```python
from build123d import *

# Parameters (mm, degrees)
SKETCH_1_W          = 92
SKETCH_1_H          = 67
EXTRUDE_1_DEPTH     = 34
SKETCH_2_W          = 86
SKETCH_2_H          = 61
CUT_EXTRUDE_1_DEPTH = 3
SKETCH_3_R          = 1.5
CUT_EXTRUDE_2_DEPTH = 3
SKETCH_4_W          = 86
SKETCH_4_H          = 61
CUT_EXTRUDE_3_DEPTH = 3
SKETCH_5_R          = 1.5
CUT_EXTRUDE_4_DEPTH = 3


with BuildPart() as part:
    # 草图1 → 凸台-拉伸1 (new body)
    with BuildSketch(Plane(origin=(0, 0, 0), x_dir=(1, 0, 0), z_dir=(0, 1, 0))):
        Rectangle(SKETCH_1_W, SKETCH_1_H)
    extrude(amount=EXTRUDE_1_DEPTH)

    # 草图2 → 切除-拉伸1 (cut)
    with BuildSketch(Plane(origin=(0, 34, 0), x_dir=(1, 0, 0), z_dir=(0, 1, 0))):
        Rectangle(SKETCH_2_W, SKETCH_2_H)
    extrude(amount=-CUT_EXTRUDE_1_DEPTH, mode=Mode.SUBTRACT)

    # 草图3 → 切除-拉伸2 (cut)
    with BuildSketch(Plane(origin=(0, 31, 0), x_dir=(1, 0, 0), z_dir=(0, 1, 0))):
        with Locations(Location((25, -16.5, 0), (0, 0, 270))):
            Circle(SKETCH_3_R)
        with Locations(Location((25, -7.5, 0), (0, 0, 270))):
            Circle(SKETCH_3_R)
    extrude(amount=-CUT_EXTRUDE_2_DEPTH, mode=Mode.SUBTRACT)

    # 草图4 → 切除-拉伸3 (cut)
    with BuildSketch(Plane.XZ):
        Rectangle(SKETCH_4_W, SKETCH_4_H)
    extrude(amount=-CUT_EXTRUDE_3_DEPTH, mode=Mode.SUBTRACT)

    # 草图5 → 切除-拉伸4 (cut)
    with BuildSketch(Plane.XZ.offset(-3)):
        with Locations(Location((-39, 24.5, 0), (0, 0, 270))):
            Circle(SKETCH_5_R)
        with Locations(Location((19, 24.5, 0), (0, 0, 90))):
            Circle(SKETCH_5_R)
        with Locations(Location((19, -24.5, 0), (0, 0, 270))):
            Circle(SKETCH_5_R)
        with Locations(Location((-39, -24.5, 0), (0, 0, 90))):
            Circle(SKETCH_5_R)
    extrude(amount=-CUT_EXTRUDE_4_DEPTH, mode=Mode.SUBTRACT)


solid = part.part
```
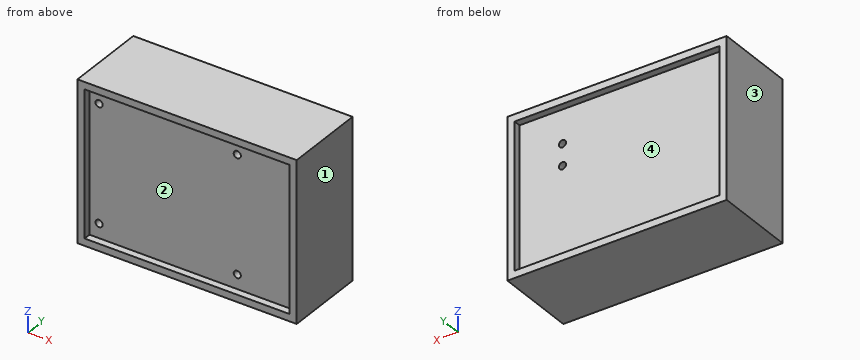
Build history of the part. All positions in model axes, mm. Face numbers are marked on the shaded views. Give positions to 0.01 mm unless a question says otherwise; leave off trailing zeros. Loops run counter-clockwise (first coordinate to the right, second up) from the corner with the lowest first, then second, coordinate; pieces in that order, holes last.
Item 1: Slice it at A-A, the plane z = -29. List the corners of the cut face in (x, y), and give its area (3 significant figures).
Answers follow:
outline: (-46, 0) - (-43, 0) - (-43, 3) - (43, 3) - (43, 0) - (46, 0) - (46, 34) - (43, 34) - (43, 31) - (-43, 31) - (-43, 34) - (-46, 34) - close
area: 2,610 mm2
Item 2: Flat gauge pins, fed straight in: pin 1 (1.5 mm diameter, centred on x = 28.5, z = 10, fed in from -Y); pin 2 (3.5 mm diameter, centred on x = -39, z = 24.5, fed in from +Y); pin 3 (0.9 mm diameter, centred on x = 19.5, z = -24, fed in from -Y). Where does each tip first touch, or does it go through?
Answers follow:
pin 1: stops at y = 3
pin 2: stops at y = 31
pin 3: stops at y = 6
Item 3: Slice it at B-B, the plane x = 6. List the corners of the cut face in (y, z).
Answers follow:
outline: (0, -33.5) - (34, -33.5) - (34, -30.5) - (31, -30.5) - (31, 30.5) - (34, 30.5) - (34, 33.5) - (0, 33.5) - (0, 30.5) - (3, 30.5) - (3, -30.5) - (0, -30.5) - close
Item 4: Slice it at C-C, the plane z = 16.5. List the corners of the cut face in (x, y), and give its area (3 significant figures).
Answers follow:
outline: (-46, 0) - (-43, 0) - (-43, 3) - (43, 3) - (43, 0) - (46, 0) - (46, 34) - (43, 34) - (43, 31) - (26.5, 31) - (26.5, 28) - (23.5, 28) - (23.5, 31) - (-43, 31) - (-43, 34) - (-46, 34) - close
area: 2,600 mm2
Item 5: Pull direction X, two halves, no side cores. Call the marked faces 1, 2, 3 and 4: released by +X, released by -X, zero draft, split by the parting line, or undercut.
Answers follow:
face 1: released by +X
face 2: undercut
face 3: released by -X
face 4: undercut
Item 6: Slice it at D-D, the plane x = -39. List the corners of the cut face in (y, z), and give its area (3 significant figures).
Answers follow:
outline: (0, -33.5) - (34, -33.5) - (34, -30.5) - (31, -30.5) - (31, 30.5) - (34, 30.5) - (34, 33.5) - (0, 33.5) - (0, 30.5) - (3, 30.5) - (3, 26) - (6, 26) - (6, 23) - (3, 23) - (3, -23) - (6, -23) - (6, -26) - (3, -26) - (3, -30.5) - (0, -30.5) - close
area: 1,890 mm2
Item 7: Drill centre lines: line 1 (X direction, y = 4.25, z = -24.5); line 2 (Z direction, x = 24.5, y = 32); line 3 (X direction, y = 28.85, z = 7.5). Where is each one in solid material? Low to high.
Answers follow:
line 1: x = -46 to -40.5, -37.5 to 17.5, 20.5 to 46
line 2: z = -33.5 to -30.5, 30.5 to 33.5
line 3: x = -46 to 23.5, 26.5 to 46
